from build123d import *

# Parameters (mm, degrees)
SKETCH1_W                    = 5.7
SKETCH1_H                    = 4.1
BOSS_EXTRUDE1_DEPTH          = 1.8
SKETCH3_R                    = 0.425
BOSS_EXTRUDE3_DEPTH          = 2.5
FILLET2_R                    = 0.425
M1_2X0_25_TAPPED_HOLE1_D     = 0.95
M1_2X0_25_TAPPED_HOLE1_DEPTH = 3.15
M1_2X0_25_TAPPED_HOLE1_TIP   = 0.285408794


with BuildPart() as part:
    # Sketch1 → Boss-Extrude1 (new body)
    with BuildSketch(Plane(origin=(0, 0, 0), x_dir=(1, 0, 0), z_dir=(0, 1, 0))):
        with Locations((2.85, -2.05)):
            Rectangle(SKETCH1_W, SKETCH1_H)
    extrude(amount=-BOSS_EXTRUDE1_DEPTH)

    # Sketch3 → Boss-Extrude3 (add)
    with BuildSketch(Plane(origin=(5.7, 0, 0), x_dir=(0, 0, -1), z_dir=(1, 0, 0))):
        with Locations((-2.05, -0.54)):
            Circle(SKETCH3_R)
    extrude(amount=BOSS_EXTRUDE3_DEPTH)

    # Fillet2
    fillet2_edges = [part.edges().sort_by_distance(p)[0] for p in [
        (8.2, -0.54, 2.475),
    ]]
    fillet(fillet2_edges, radius=FILLET2_R)

    # M1.2x0.25 Tapped Hole1
    with Locations(Plane(origin=(0, -1.8, 0), x_dir=(-1, 0, 0), z_dir=(0, -1, 0))):
        with Locations((-4.45, -2.05), (-1.45, -2.05)):
            Hole(M1_2X0_25_TAPPED_HOLE1_D / 2, depth=M1_2X0_25_TAPPED_HOLE1_DEPTH)
            with Locations((0, 0, -(M1_2X0_25_TAPPED_HOLE1_DEPTH + M1_2X0_25_TAPPED_HOLE1_TIP / 2))):  # 118° drill point
                Cone(0, M1_2X0_25_TAPPED_HOLE1_D / 2, M1_2X0_25_TAPPED_HOLE1_TIP, mode=Mode.SUBTRACT)


solid = part.part
Design review of the part built by this model. Coordinates are the model's own, in mm. Round coordinates to 2 decimals unless told otherwise and drop trailing zeros. Write each loop counter-clockwise with the first axis right and the second up, starting at its lowest first coordinate (ties: lowest second). Pieces come first, ordered by that corner, then holes. Notation, with made-up numbers: M -34.75,64.5 L 1.25,64.5 A9 ccw 1.25,74.5 Z; hole C -10.75,83.25 d11. An arc over 180 degrees is marked long. One line per item, written item: value. Start each with the question number.
1. Take a section at A-A on z = 2.05. State the section outline as (x, y) points (3 decimals).
2. Take a section at C-C on y = -0.54. State the section outline as (x, z) points (3 decimals).
3. To check wall thickness, follow probe 1 along Z at (x, y) = (4.45, -0.65) (3 decimals); probe 2 along X at (y, z) = (-1.25, 2.05) (3 decimals); probe 3 along X at (y, z) = (-0.35, 2.05) (3 decimals). State the ranges of each line that lie inside material, in increasing order. Write a range as from..to.
4. Draft analysis for pull direction X (two halves, no side actions). For faces 1 (the face through (4.67, -0.89, 2.47)), 2 (the face through (5.7, -1.3, 2.1)), 3 (the face through (6.723, -0.412, 1.645)), state which applies: pulls with the +X half, pulls with the -X half, needs draft (parallel to the pull), parting line crosses it, or undercut.
5. Take a section at D-D on x = 7. State the section outline as (y, z) points (3 decimals).
6. Take a section at B-B on x = 4.45. State the section outline as (y, z) points (3 decimals).
Computed:
1. outline: M 0,-1.8 L 0.975,-1.8 L 0.975,0 L 0,0 Z; M 1.925,-1.8 L 3.975,-1.8 L 3.975,0 L 1.925,0 Z; M 4.925,-1.8 L 5.7,-1.8 L 5.7,-0.965 L 7.775,-0.965 A0.425 ccw 7.775,-0.115 L 5.7,-0.115 L 5.7,0 L 4.925,0 Z
2. outline: M 0,0 L 5.7,0 L 5.7,1.625 L 7.775,1.625 A0.425 ccw 7.775,2.475 L 5.7,2.475 L 5.7,4.1 L 0,4.1 Z; hole C 1.45,2.05 d0.95; hole C 4.45,2.05 d0.95
3. probe 1: z = 0..1.575, 2.525..4.1
3. probe 2: x = 0..0.975, 1.925..3.975, 4.925..5.7
3. probe 3: x = 0..0.975, 1.925..3.975, 4.925..8.155
4. face 1: undercut
4. face 2: pulls with the +X half
4. face 3: needs draft
5. outline: C -0.54,2.05 d0.85
6. outline: M -1.8,0 L 0,0 L 0,1.575 L -1.8,1.575 Z; M -1.8,2.525 L 0,2.525 L 0,4.1 L -1.8,4.1 Z
